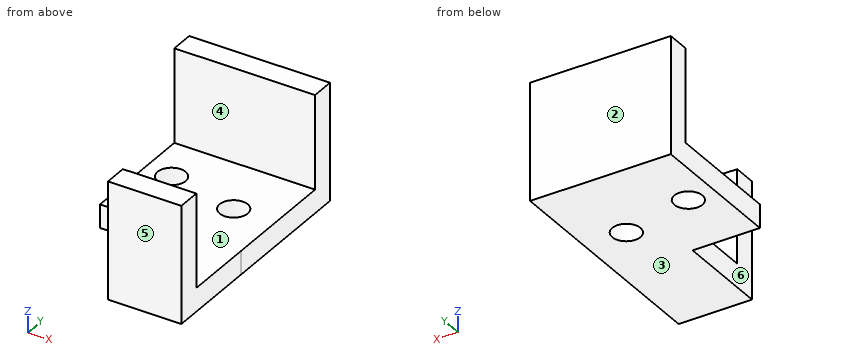
from build123d import *

# Parameters (mm, degrees)
F0_W     = 152.4
F0_H     = 25.4
F1_DEPTH = 127
F0_R     = 15.24
F0_W_2   = 79.522247
F0_H_2   = 76.2
F2_DEPTH = 25.4
F3_DEPTH = 127


with BuildPart() as f1:
    # F0 (on Top) → F1 (new body)
    with BuildSketch(Plane.XY):
        with Locations((3.322247, 63.5)):
            Rectangle(F0_W, F0_H)
    extrude(amount=F1_DEPTH)

    # F0 (on Top) → F2 (join)
    with BuildSketch(Plane.XY):
        Polygon((79.522247, 50.8), (-72.877753, 50.8), (-72.877753, -76.2), (0, -76.2), (79.522247, -76.2), align=None)
        with Locations((-43.653723, 0)):
            Circle(F0_R, mode=Mode.SUBTRACT)
        with Locations((34.601994, -17.455092)):
            Circle(F0_R, mode=Mode.SUBTRACT)
        with Locations((39.761123, -114.3)):
            Rectangle(F0_W_2, F0_H_2)
    extrude(amount=F2_DEPTH)

    # F0 (on Top) → F3 (join)
    with BuildSketch(Plane.XY):
        with Locations((39.761123, -165.1)):
            Rectangle(F0_W_2, F0_H)
    extrude(amount=F3_DEPTH)


solid = f1.part
Can you work these out from the model? Positions are in its coordinate system, mm. Face numbers are marked on the shaded views. A direction names the side the tool comes from. Coordinates: 2 decimals unless noted, no trailing zeros. Loops run counter-clockwise (first coordinate to the right, second up) from the corner with the lowest first, then second, coordinate; pieces in that order, holes last. Notation, with made-up numbers: (-9.75, 4) - (38.25, 4) arc R17 cw to (38.25, 11) - close; hole circle Ø10 at (15.25, -2.75). An arc over 180 degrees is marked (long way). Put each result on its own line as item: value. Start each with the question number.
Item 1: Which directions (+Z, -Z, +X, -X, +Y, -Y) give clear straight access to the entire face, cutting with the end or side of a thin tool? Please do the marked faces 5 and 6.
Item 2: Suppose I cut it at D-D (y = -67). Please give me the cut outline in (x, z).
Item 3: Suppose I cut it at B-B (x = -21.5). Please give me the cut outline in (y, z).
Item 4: If we mould it in two halves opening along Y, with no side actions, what happens to the marked faces 1, 2, 3 and 4? For each: +Y half, -Y half, draft (parallel to the pull), parting line (faces both ways), or undercut.
Item 5: If I drill on line 1 along Y through (x, z) = (-63, 6); line 2 along Y through (x, z) = (-27.5, 61); line 3 along Z through (x, y) = (-64, 40), over which ranges is the centre line in solid material (lowest first)?
Item 6: Suppose I cut it at A-A (z = 108.5). Please give me the cut outline in (x, y).
Item 7: For pin 1 (20.5 mm diameter, centred on x = -51, z = 18.5, fed in from -Y), with a flat end and sliding along its axis, tell me the tip position at first contact or that it passes through.
Item 8: Suppose I cut it at C-C (y = -30). Please give me the cut outline in (x, z), and give its area (3 significant figures).
Here are the results:
1. face 5: +Z, -Z, +X, -X, -Y
1. face 6: +Z, -Z, -X, -Y
2. outline: (-72.88, 0) - (79.52, 0) - (79.52, 25.4) - (-72.88, 25.4) - close
3. outline: (-76.2, 0) - (76.2, 0) - (76.2, 127) - (50.8, 127) - (50.8, 25.4) - (-76.2, 25.4) - close
4. face 1: undercut
4. face 2: +Y half
4. face 3: draft
4. face 4: undercut
5. line 1: -76.2 to 76.2
5. line 2: 50.8 to 76.2
5. line 3: 0 to 25.4
6. outline: (-72.88, 50.8) - (79.52, 50.8) - (79.52, 76.2) - (-72.88, 76.2) - close; (0, -177.8) - (79.52, -177.8) - (79.52, -152.4) - (0, -152.4) - close
7. pin 1: y = -76.2
8. outline: (-72.88, 0) - (25.95, 0) - (25.95, 25.4) - (-72.88, 25.4) - close; (43.26, 0) - (79.52, 0) - (79.52, 25.4) - (43.26, 25.4) - close
8. area: 3,430 mm²
